The model under review builds one solid part; all positions refer to its coordinate system, in mm. A direction names the side the tool comes from. Coordinates: 2 decimals unless noted, no trailing zeros. Order: outer loops, then holes, each group sorted by start corner. A loop starts at its lowest first (then second) coordinate and runs counter-clockwise, first axis right, second up. Notation, with made-up numbers: (29, 57) - (38, 57) arc R23 cw to (38, 70) - close; hole circle Ø5 at (29, 87.5). An arc over 180 degrees is marked (long way). Answer in a Markdown table with one row per item.
Autodesk Inventor part; units mm, degrees
ref_plane "bearings_XY" through (0, 0, 0) normal (0, 0, 1) x (1, 0, 0)
ref_plane "bearings_YZ" through (0, 0, 0) normal (1, 0, 0) x (0, 1, 0)
ref_plane "bearings_ZX" through (0, 0, 0) normal (0, 1, 0) x (0, 0, 1)
sketch "Sketch_2" plane through (0, 0, 0) normal (1, 0, 0) x (0, 1, 0)
  line L0 (0, -13.0048) -> (0, 2.6162)
  line L1 (8.7847, 2.6162) -> (6.6294, 0.4609)
  line L2 (6.6294, 0.4609) -> (6.6294, -10.8495)
  line L3 (6.6294, -10.8495) -> (8.7847, -13.0048)
  line L4 (8.7847, -13.0048) -> (10.4159, -13.0048)
  line L5 (10.4159, -13.0048) -> (11.4935, -11.9272)
  line L6 (11.4935, -11.9272) -> (11.4935, 0)
  line L7 (11.4935, 0) -> (13.462, 0)
  line L8 (13.462, 0) -> (13.462, 2.6162)
  line L9 (13.462, 2.6162) -> (8.7847, 2.6162)
revolve "Revolution1" add sketch "Sketch_2" angle 360 about axis through (0, 0, -13.0048) along (0, 0, -1)
ref_plane "bearings_XY" through (0, 0, 0) normal (0, 0, 1) x (1, 0, 0)
ref_plane "bearings_YZ" through (0, 0, 0) normal (1, 0, 0) x (0, 1, 0)
ref_plane "bearings_ZX" through (0, 0, 0) normal (0, 1, 0) x (0, 0, 1)
ref_plane "to_washer1_XY" through (0, 0, 0) normal (0, 0, 1) x (1, 0, 0)
ref_plane "to_washer1_YZ" through (0, 0, 0) normal (1, 0, 0) x (0, 1, 0)
ref_plane "to_washer1_ZX" through (0, 0, 0) normal (0, 1, 0) x (0, 0, 1)
ref_plane "to_washer2_XY" through (0, 0, 0) normal (0, 0, 1) x (1, 0, 0)
ref_plane "to_washer2_YZ" through (0, 0, 0) normal (1, 0, 0) x (0, 1, 0)
ref_plane "to_washer2_ZX" through (0, 0, 0) normal (0, 1, 0) x (0, 0, 1)
properties part number "52008.48"
Item 1: We need section C-C, the plane z = -0.75. Write out the cut boundary in (x, y).
Check values:
| item | result |
|---|---|
| outline | circle Ø22.99 at (0, 0); hole circle Ø13.26 at (0, 0) |
Item 2: Clearance check with flat-ended pins moving along their axes: pin 1 Ø5 at (x, z) = (-2.5, -1.5) entering from +Y; pin 2 Ø8 at (x, y) = (2, -5.5) entering from +Z; pin 3 Ø5 at (x, y) = (-3.5, -2.5) entering from +Z; pin 4 Ø8 at (x, z) = (9.5, -5) entering from -Y. State where each tip first meets the part, or that it passes through.
Check values:
| item | result |
|---|---|
| pin 1 | y = 13.45 |
| pin 2 | z = 2.62 |
| pin 3 | z = 0.63 |
| pin 4 | y = -10.09 |
Item 3: To check wall thickness, follow line 1 (X direction, y = 0, z = -8); line 2 (Z direction, x = -6, y = 10.5); line 3 (X direction, y = -4.75, z = 1.5). State the ranges of each line that lie inside material, in increasing order. Write a range as from..to.
Check values:
| item | result |
|---|---|
| line 1 | -11.49..-6.63, 6.63..11.49 |
| line 2 | 0..2.62 |
| line 3 | -12.6..-6.02, 6.02..12.6 |
Item 4: We need section A-A, the plane x = 0. Write out the cut boundary in (y, z), then the cut area to 3 significant figures.
Check values:
| item | result |
|---|---|
| outline | (-13.46, 0) - (-11.49, 0) - (-11.49, -11.93) - (-10.42, -13) - (-8.78, -13) - (-6.63, -10.85) - (-6.63, 0.46) - (-8.78, 2.62) - (-13.46, 2.62) - close; (6.63, -10.85) - (8.78, -13) - (10.42, -13) - (11.49, -11.93) - (11.49, 0) - (13.46, 0) - (13.46, 2.62) - (8.78, 2.62) - (6.63, 0.46) - close |
| area | 152 mm^2 |
Item 5: Tool access review of faces 1 (the face through (6, 10, 0)), 2 (the face through (8.191, -10.683, 1.326)): name each direction out of +Z, -Z, +X, -X, +Y, -Y from which nothing blocks a thin tool from reaching the whole face with its end or side.
Check values:
| item | result |
|---|---|
| face 1 | -Z |
| face 2 | +Z, -Z |
